Model file for the job. Use its own axes, mm. Give positions to 0.01 mm unless a question says otherwise; leave off trailing zeros. Write each loop counter-clockwise with the first axis right and the second up, starting at its lowest first coordinate (ties: lowest second). Pieces come first, ordered by that corner, then holes. Notation, with made-up numbers: (83.25, 25) - (127.25, 25) arc R14 ccw to (127.25, 50) - close; hole circle Ø8 at (-33.5, 73). An arc over 180 degrees is marked (long way). One line per item, written item: value. Start each with the question number.
(1) Probe L1, parallel to Z at x = -470.5, y = 0 (1 decimal); L2, parallel to Y at x = -238, z = -1.25; L3, parallel to Y at x = -298, z = -0.5. List the from-to ranges inside material, lowest first.
(2) Drop flat-ended pins along their axis: P1, Ø1, axis at x = 143.5, y = 5, coming from the -Z side; P2, Ø1.5, axis at x = -207.5, z = -3, coming from the -Y side; P3, Ø5.5, axis at y = 0, z = 0, coming from the -X side. Give the stop position or say it passes through.
(3) Cut at A-A, the plane x = 290.5. List the corners of the cut face in (y, z) (1 decimal).
from build123d import *

# Parameters (mm, degrees)
F0_R           = 7.9375
F1_DEPTH       = 479.425
F3_D           = 6.35
F3_DEPTH       = 25.4
F3_CSINK_D     = 7.62
F3_CSINK_ANGLE = 90
F3_TIP         = 1.9077324654
F5_D           = 6.35
F5_DEPTH       = 25.4
F5_CSINK_D     = 7.62
F5_CSINK_ANGLE = 90
F5_TIP         = 1.9077324654


with BuildPart() as f1:
    # F0 (on Right) → F1 (new body, symmetric)
    with BuildSketch(Plane.YZ):
        Circle(F0_R)
    extrude(amount=F1_DEPTH, both=True)

    # F3
    with Locations(Plane(origin=(-479.425, 0, 0), x_dir=(0, -1, 0), z_dir=(-1, 0, 0))):
        with Locations((0, 0)):
            CounterSinkHole(F3_D / 2, F3_CSINK_D / 2, depth=F3_DEPTH, counter_sink_angle=F3_CSINK_ANGLE)
            with Locations((0, 0, -(F3_DEPTH + F3_TIP / 2))):  # 118° drill point
                Cone(0, F3_D / 2, F3_TIP, mode=Mode.SUBTRACT)

    # F5
    with Locations(Plane.YZ.offset(479.425)):
        with Locations((0, 0)):
            CounterSinkHole(F5_D / 2, F5_CSINK_D / 2, depth=F5_DEPTH, counter_sink_angle=F5_CSINK_ANGLE)
            with Locations((0, 0, -(F5_DEPTH + F5_TIP / 2))):  # 118° drill point
                Cone(0, F5_D / 2, F5_TIP, mode=Mode.SUBTRACT)


solid = f1.part
Answers follow:
1. L1: z = -7.9 to -3.2, 3.2 to 7.9
1. L2: y = -7.84 to 7.84
1. L3: y = -7.92 to 7.92
2. P1: stops at z = -6.54
2. P2: stops at y = -7.61
2. P3: stops at x = -453.77
3. outline: circle Ø15.9 at (0, 0)
